The model under review builds one solid part; all positions refer to its coordinate system, in mm. Give positions to 0.01 mm unless a question says otherwise; leave off trailing zeros. Order: outer loops, then holes, each group sorted by start corner. A loop starts at its lowest first (then second) coordinate and runs counter-clockwise, first axis right, second up. Notation, with made-up numbers: (-12.75, 36.5) - (-4.75, 36.5) arc R21 ccw to (-4.75, 71.5) - close; hole circle Ø2 at (22.5, -39.75). An arc over 180 degrees is marked (long way). Answer as CSV lines item,"result". Start each with the question number.
from build123d import *

# Parameters (mm, degrees)
SKETCH1_R           = 10
SKETCH1_R_2         = 1.25
SKETCH1_R_3         = 1.5
BOSS_EXTRUDE1_DEPTH = 2.5
SKETCH2_R           = 1.03251
CUT_EXTRUDE1_DEPTH  = 15.361406616


with BuildPart() as part:
    # Sketch1 → Boss-Extrude1 (new body)
    with BuildSketch(Plane(origin=(0, 0, 0), x_dir=(1, 0, 0), z_dir=(0, 1, 0))):
        with Locations(Location((0, 0, 0), (0, 0, 270))):
            Circle(SKETCH1_R)
        with Locations(Location((-8, 0, 0), (0, 0, 270))):
            Circle(SKETCH1_R_2, mode=Mode.SUBTRACT)
        with Locations(Location((0, -8, 0), (0, 0, 270))):
            Circle(SKETCH1_R_2, mode=Mode.SUBTRACT)
        with Locations(Location((8, 0, 0), (0, 0, 270))):
            Circle(SKETCH1_R_2, mode=Mode.SUBTRACT)
        with Locations(Location((0, 8, 0), (0, 0, 270))):
            Circle(SKETCH1_R_2, mode=Mode.SUBTRACT)
        with Locations(Location((0, 0, 0), (0, 0, 270))):
            Circle(SKETCH1_R_3, mode=Mode.SUBTRACT)
    extrude(amount=BOSS_EXTRUDE1_DEPTH)

    # Sketch2 → Cut-Extrude1 (cut, through all)
    with BuildSketch(Plane(origin=(0, 2.5, 0), x_dir=(1, 0, 0), z_dir=(0, 1, 0))):
        with Locations(Location((-4.041115254, 4.041115254, 0), (0, 0, 270))):
            Circle(SKETCH2_R)
        with Locations(Location((4.041115254, 4.041115254, 0), (0, 0, 270))):
            Circle(SKETCH2_R)
        with Locations(Location((4.041115254, -4.041115254, 0), (0, 0, 270))):
            Circle(SKETCH2_R)
        with Locations(Location((-4.041115254, -4.041115254, 0), (0, 0, 270))):
            Circle(SKETCH2_R)
    extrude(amount=-CUT_EXTRUDE1_DEPTH, mode=Mode.SUBTRACT)


solid = part.part
Item 1: Clearance check with flat-ended pins moving along their axes: pin 1 (3 mm diameter, centred on x = -8, z = 0, fed in from +Y); pin 2 (1.5 mm diameter, centred on x = -1.5, y = 1.5, fed in from +Z); pin 3 (2 mm diameter, centred on x = 0, z = -8, fed in from -Y); pin 4 (1 mm diameter, centred on y = 1.5, z = -1.5, fed in from +X). State where each tip first meets the part, or that it passes through.
Item 2: For line 1 along X through (y, z) = (1.2, 0); line 2 along Z through (x, y) = (0.75, 2); line 3 along X through (y, z) = (0.7, 4.5), list the stretches that pass through material, from the lowest coordinate up.
Item 3: Take a section at D-D on x = 4.5. Write out the cut boundary in (y, z), and give its area (3 significant figures).
Item 4: Mouldability with a two-part tool opening along Z and no side actions: class faces 1 (the face through (-2, 0, 0)), 2 (the face through (-9.22, 1.23, -0.27)), 3 (the face through (-9.76, 1.23, -2.17)) as released by +Z, released by -Z, zero draft, split by the parting line, or undercut.
Item 5: Take a section at B-B on x = 8. Write out the cut boundary in (y, z), and give its area (4 significant figures).
Item 6: Take a section at C-C on z = 0. Write out the cut boundary in (x, y), and give its area (3 significant figures).
Item 7: Take a section at A-A on z = -8. Write out the cut boundary in (x, y), and give its area (4 significant figures).
Data:
1,pin 1,"stops at y = 2.5"
1,pin 2,"stops at z = 9.97"
1,pin 3,"passes through"
1,pin 4,"stops at x = 9.95"
2,line 1,"x = -10 to -9.25, -6.75 to -1.5, 1.5 to 6.75, 9.25 to 10"
2,line 2,"z = -9.97 to -9, -7 to -1.3, 1.3 to 7, 9 to 9.97"
2,line 3,"x = -8.93 to -4.97, -3.12 to 3.12, 4.97 to 8.93"
3,outline,"(0, -8.93) - (2.5, -8.93) - (2.5, -4.97) - (0, -4.97) - close; (0, -3.12) - (2.5, -3.12) - (2.5, 3.12) - (0, 3.12) - close; (0, 4.97) - (2.5, 4.97) - (2.5, 8.93) - (0, 8.93) - close"
3,area,"35.4 mm^2"
4,face 1,"zero draft"
4,face 2,"undercut"
4,face 3,"split by the parting line"
5,outline,"(0, -6) - (2.5, -6) - (2.5, -1.25) - (0, -1.25) - close; (0, 1.25) - (2.5, 1.25) - (2.5, 6) - (0, 6) - close"
5,area,"23.75 mm^2"
6,outline,"(-10, 0) - (-9.25, 0) - (-9.25, 2.5) - (-10, 2.5) - close; (-6.75, 0) - (-1.5, 0) - (-1.5, 2.5) - (-6.75, 2.5) - close; (1.5, 0) - (6.75, 0) - (6.75, 2.5) - (1.5, 2.5) - close; (9.25, 0) - (10, 0) - (10, 2.5) - (9.25, 2.5) - close"
6,area,"30.0 mm^2"
7,outline,"(-6, 0) - (-1.25, 0) - (-1.25, 2.5) - (-6, 2.5) - close; (1.25, 0) - (6, 0) - (6, 2.5) - (1.25, 2.5) - close"
7,area,"23.75 mm^2"
